Can you work these out from the model? Positions are in its coordinate system, mm. A direction names the side the tool comes from. Coordinates: 2 decimals unless noted, no trailing zeros. Order: outer loops, then holes, each group sorted by start corner. A loop starts at its lowest first (then second) coordinate and runs counter-clockwise, first axis right, second up. Notation, with made-up numbers: (56.5, 56) -> (85.5, 56) arc R18 ccw to (85.5, 65) -> close; hole circle Ø8 at (-35, 5.5). An arc over 180 degrees is marked (long way). Answer in a Markdown table with one row per item.
```python
from build123d import *

# Parameters (mm, degrees)
F0_W     = 10
F0_H     = 15.588
F1_DEPTH = 20
F2_W     = 10
F2_H     = 15.588
F3_DEPTH = 23
F5_DEPTH = 15.589
F6_DEPTH = 15.589


with BuildPart() as f1:
    # F0 (on Top) → F1 (new body)
    with BuildSketch(Plane.XY):
        Polygon((-20.4545138283, 3.49999999), (-19.7328258911, 4.7500001644), (-17.9753717666, 7.794), (-22.9753717666, 7.794), (-22.9753717666, -7.794), (-17.9753717666, -7.794), (-19.732826028, -4.7499999273), (-20.4545138514, -3.49999995), (-22.4752397647, 0), align=None)
        with Locations((-27.9753717666, 0)):
            Rectangle(F0_W, F0_H)
    extrude(amount=F1_DEPTH)

    # F2 (on face) → F3 (join)
    with BuildSketch(Plane.XY.offset(20)):
        with Locations((-27.9753717666, 0)):
            Rectangle(F2_W, F2_H)
    extrude(amount=F3_DEPTH)

    # F4 (on face) → F5 (cut, through all)
    with BuildSketch(Plane.XZ.offset(7.794)):
        Polygon((-32.9753717666, 0), (-28.9753717666, 0), (-28.9753717666, 20), (-28.9753717666, 30.5), (-32.9753717666, 30.5), align=None)
    extrude(amount=-F5_DEPTH, mode=Mode.SUBTRACT)

    # F4 (on face) → F6 (cut, through all)
    with BuildSketch(Plane.XZ.offset(7.794)):
        Polygon((-28.9753717666, 0), (-20.9753717666, 0), (-28.9753717666, 20), align=None)
    extrude(amount=-F6_DEPTH, mode=Mode.SUBTRACT)


solid = f1.part
```
(1) On a 3-axis mill with a long thin cutter (end or side, diameter ignored), from which of +Z, -Z, +X, -X, +Y, -Y can I reach the whole of each face in a straight line? I mean faces 1 (the flat face through (-22.7, 0.1, 20)), 2 (the flat face through (-28.975, 0, 25)), 3 (the flat face through (-26, 7.794, 26)). Say none if no direction works.
Response values:
| item | result |
|---|---|
| face 1 | +Z, +X, +Y, -Y |
| face 2 | -Z, -X, +Y, -Y |
| face 3 | +Z, -Z, +X, -X, +Y |
(2) Suppose I cut it at C-C (y = 0.5). Please give me the cut outline in (x, z), and give its area (3 significant figures).
Response values:
| item | result |
|---|---|
| outline | (-32.98, 30.5) -> (-28.98, 30.5) -> (-28.98, 20) -> (-22.19, 3.03) -> (-22.19, 20) -> (-22.98, 20) -> (-22.98, 43) -> (-32.98, 43) -> close |
| area | 246 mm2 |
(3) Suppose I cut it at B-B (z = 16). Please give me the cut outline in (x, y).
Response values:
| item | result |
|---|---|
| outline | (-27.38, -7.79) -> (-17.98, -7.79) -> (-22.48, 0) -> (-17.98, 7.79) -> (-27.38, 7.79) -> close |
(4) Will these pins go through, and if not, where does the flat tip stop? pin 1 Ø1 at (y, z) = (-5, 20) entering from -X; pin 2 Ø2 at (y, z) = (-2.5, 10.5) entering from +X; pin 3 Ø1.5 at (x, y) = (-21, -3.5) entering from +Z.
Response values:
| item | result |
|---|---|
| pin 1 | x = -28.98 |
| pin 2 | x = -20.45 |
| pin 3 | z = 20 |
(5) Suppose I cut it at D-D (x = -30). Please give me the cut outline in (y, z), and give its area (3 significant figures).
Response values:
| item | result |
|---|---|
| outline | (-7.79, 30.5) -> (7.79, 30.5) -> (7.79, 43) -> (-7.79, 43) -> close |
| area | 195 mm2 |
(6) Suppose I cut it at A-A (x = -22). Please give me the cut outline in (y, z), and give its area (3 significant figures).
Response values:
| item | result |
|---|---|
| outline | (-7.79, 2.56) -> (-0.82, 2.56) -> (-0.82, 20) -> (-7.79, 20) -> close; (0.82, 2.56) -> (7.79, 2.56) -> (7.79, 20) -> (0.82, 20) -> close |
| area | 243 mm2 |
(7) I need wall thicknesses on line 1 (Z direction, x = -20.5, y = -6.75); line 2 (X direction, y = 1, z = 32); line 3 (Y direction, x = -21, z = 17). Which ranges of each line are inside material? Lowest first, please. Write a range as [from, to].
Response values:
| item | result |
|---|---|
| line 1 | [0, 20] |
| line 2 | [-32.98, -22.98] |
| line 3 | [-7.79, -2.56], [2.56, 7.79] |
